Source: CAD feature listing. Evaluate the final solid. Frame: model axes, mm. Round coordinates to 2 decimals unless told otherwise and drop trailing zeros. Order: outer loops, then holes, each group sorted by start corner. A loop starts at its lowest first (then second) coordinate and runs counter-clockwise, first axis right, second up. Notation, with made-up numbers: (30.25, -33.5) - (38.25, -33.5) arc R21 ccw to (38.25, -18.5) - close; hole circle Ø11 at (39, -31.5). An arc over 180 degrees is marked (long way). Use one line per item in the form item = value. Start each with the question number.
Q1. Cut plane C-C, the plane x = 8. Return the cut outline in (y, z), and give its area (3 significant figures).
Q2. Ray query, line 1 (X direction, y = 5.5, z = 12.7) (3 decimals); line 2 (X direction, y = 6, z = -64) (3 decimals); line 3 (Z direction, x = 5, y = 6.25). Return the intervals inside material, ascending. Write a range as [from, to].
Q3. Cut plane B-B, the plane x = -7. Return the cut outline in (y, z), and give its area (3 significant figures).
Q4. Cut plane A-A, the plane y = 3. Give the number of separate pieces and of enclosed holes in the cut face, and give its area (3 significant figures).
Q5. Pin query (flat end, axial travel): pin 1 Ø2 at (x, z) = (0, -38.1) entering from -Y; pin 2 Ø3.5 at (x, z) = (0, -12.7) entering from -Y. Return the tip coordinate at first contact, or that it passes through.
Autodesk Inventor part; units mm, degrees
ref_plane "YZ Plane" through (0, 0, 0) normal (1, 0, 0) x (0, 1, 0)
ref_plane "XZ Plane" through (0, 0, 0) normal (0, 1, 0) x (-1, 0, 0)
ref_plane "XY Plane" through (0, 0, 0) normal (0, 0, 1) x (1, 0, 0)
sketch "Sketch1" plane through (0, 0, 0) normal (0, 1, 0) x (-1, 0, 0)
  line L0 (0, -88.9) -> (0, 88.9) construction
  line L1 (15.875, -88.9) -> (15.875, 88.9)
  line L2 (-15.875, 88.9) -> (-15.875, -88.9)
  arc A0 (-15.875, -88.9) -> (15.875, -88.9) centre (0, -88.9) ccw
  arc A1 (15.875, 88.9) -> (-15.875, 88.9) centre (0, 88.9) ccw
  point P0 (0, 0)
  point P1 (0, 63.5)
  point P2 (0, 38.1)
  point P3 (0, 12.7)
  point P4 (0, -12.7)
  point P5 (0, -38.1)
  point P6 (0, -63.5)
  point P7 (0, -88.9)
  dimension "d0" = 31.75
  dimension "d1" = 177.8
  dimension "d4" = 25.4
extrude "Extrusion1" add sketch "Sketch1" along normal blind 7.62
hole "Hole1" at (0, 0, 88.9) at (0, 0, 63.5) at (0, 0, 38.1) at (0, 0, 12.7) at (0, 0, -12.7) at (0, 0, -38.1) at (0, 0, -63.5) at (0, 0, -88.9) direction (0, 1, 0) diameter 2.54 end through all
Completed:
q1.outline = (0, -102.61) - (7.62, -102.61) - (7.62, 102.61) - (0, 102.61) - close
q1.area = 1,560 mm2
q2.line_1 = [-15.875, -1.27], [1.27, 15.875]
q2.line_2 = [-15.875, -1.167], [1.167, 15.875]
q2.line_3 = [-103.97, 103.97]
q3.outline = (0, -103.15) - (7.62, -103.15) - (7.62, 103.15) - (0, 103.15) - close
q3.area = 1,570 mm2
q4.separate_pieces = 1
q4.enclosed_holes = 8
q4.area = 6,400 mm2
q5.pin_1 = through
q5.pin_2 = 0
